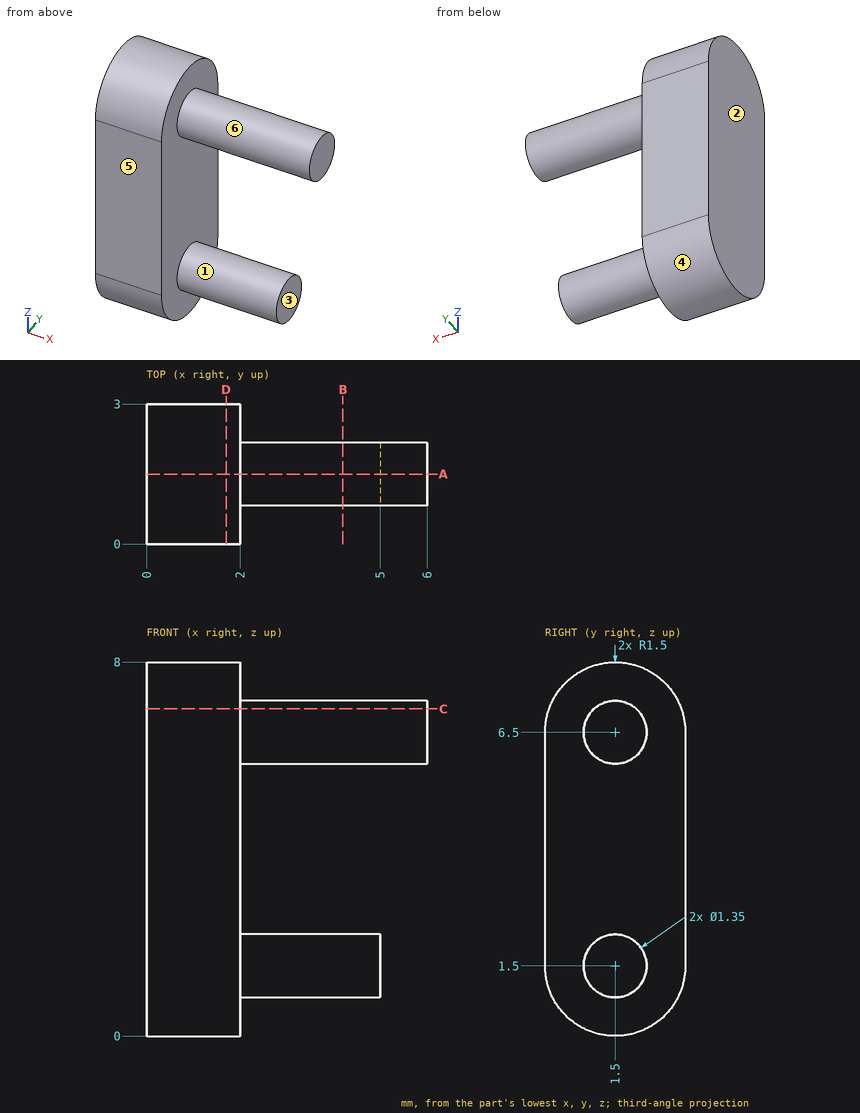
Can you work these out from the drawing? Everything is in mm from the part's minimum corner. A direction names the side the tool comes from. Coordinates: 2 decimals unless noted, no trailing zeros. Write each loop counter-clockwise with the first axis right and the second up, starting at its lowest first coordinate (ties: lowest second). Pieces come first, ordered by that corner, then holes. Notation, with made-up numbers: (32, 86) -> (89, 86) arc R20 cw to (89, 111) -> close; hole circle Ø10 at (75.25, -21.75). An arc over 180 degrees is marked (long way). Return JSON: item names as keys, results as strings.
(1) I need wall thicknesses on L1, parallel to Z at x = 4.35, y = 1.55; L2, parallel to X at y = 2.4, z = 5; L3, parallel to Z at x = 4.3, y = 1.3. Which ranges of each line are inside material? Lowest first, please.
Numbers:
{"L1": "z = 0.83 to 2.17, 5.83 to 7.17", "L2": "x = 0 to 2", "L3": "z = 0.86 to 2.14, 5.86 to 7.14"}
(2) Imagine slicing it at D-D, the plane x = 1.7. Please give me the cut outline in (y, z).
Numbers:
{"outline": "(0, 1.5) arc R1.5 ccw to (3, 1.5) -> (3, 6.5) arc R1.5 ccw to (0, 6.5) -> close"}
(3) Imagine slicing it at C-C, the plane z = 7. Please give me the cut outline in (x, y), then the cut area to 3 significant figures.
Numbers:
{"outline": "(0, 0.09) -> (2, 0.09) -> (2, 1.05) -> (6, 1.05) -> (6, 1.95) -> (2, 1.95) -> (2, 2.91) -> (0, 2.91) -> close", "area": "9.28 mm2"}
(4) I'm going to push flat-ended pins straight in: pin 1 (1 mm diameter, centred on x = 2, z = 5, fed in from -Y); pin 2 (1.5 mm diameter, centred on y = 1, z = 3.5, fed in from +X); pin 3 (3 mm diameter, centred on x = 5, z = 6, fed in from +Y) (3 decimals); pin 4 (1.1 mm diameter, centred on y = 1.5, z = 2, fed in from +X). Where does each tip first touch, or does it pass through?
Numbers:
{"pin 1": "stops at y = 0", "pin 2": "stops at x = 2", "pin 3": "stops at y = 2.175", "pin 4": "stops at x = 5"}
(5) Imagine slicing it at B-B, the plane x = 4.2. Please give me the cut outline in (y, z) (3 decimals).
Numbers:
{"outline": "circle Ø1.35 at (1.5, 1.5); circle Ø1.35 at (1.5, 6.5)"}
(6) Which directions (+Z, -Z, +X, -X, +Y, -Y) give clear straight access to the entire face, cutting with the end or side of a thin tool? Please do the marked faces 1, 2 and 3.
Numbers:
{"face 1": "+X", "face 2": "+Z, -Z, -X, +Y, -Y", "face 3": "-Z, +X, +Y, -Y"}
(7) We'd pull the mould along Z, two halves only. Please class the marked faces 4, 5 and 6: +Z half, -Z half, draft (parallel to the pull), parting line (faces both ways), or undercut.
Numbers:
{"face 4": "-Z half", "face 5": "draft", "face 6": "undercut"}
(8) Imagine slicing it at A-A, the plane y = 1.5. Please give me the cut outline in (x, z) (3 decimals).
Numbers:
{"outline": "(0, 0) -> (2, 0) -> (2, 0.825) -> (5, 0.825) -> (5, 2.175) -> (2, 2.175) -> (2, 5.825) -> (6, 5.825) -> (6, 7.175) -> (2, 7.175) -> (2, 8) -> (0, 8) -> close"}
